```python
from build123d import *

# Parameters (mm, degrees)
SKETCH1_W           = 101.4
SKETCH1_H           = 92.5
SKETCH1_R           = 1.5
SKETCH1_R_2         = 2
BOSS_EXTRUDE1_DEPTH = 10


with BuildPart() as part:
    # Sketch1 → Boss-Extrude1 (new body)
    with BuildSketch(Plane(origin=(0, 0, 0), x_dir=(1, 0, 0), z_dir=(0, 1, 0))):
        Rectangle(SKETCH1_W, SKETCH1_H)
        with Locations((-40, 42.75)):
            Circle(SKETCH1_R, mode=Mode.SUBTRACT)
        with Locations((-20, 42.75)):
            Circle(SKETCH1_R, mode=Mode.SUBTRACT)
        with Locations((-20, 17.75)):
            Circle(SKETCH1_R, mode=Mode.SUBTRACT)
        with Locations((-40, 17.75)):
            Circle(SKETCH1_R, mode=Mode.SUBTRACT)
        with Locations((-40, -42.75)):
            Circle(SKETCH1_R, mode=Mode.SUBTRACT)
        with Locations((-20, -42.75)):
            Circle(SKETCH1_R, mode=Mode.SUBTRACT)
        with Locations((-20, -17.75)):
            Circle(SKETCH1_R, mode=Mode.SUBTRACT)
        with Locations((-40, -17.75)):
            Circle(SKETCH1_R, mode=Mode.SUBTRACT)
        with Locations((40, -17.75)):
            Circle(SKETCH1_R, mode=Mode.SUBTRACT)
        with Locations((20, -17.75)):
            Circle(SKETCH1_R, mode=Mode.SUBTRACT)
        with Locations((20, -42.75)):
            Circle(SKETCH1_R, mode=Mode.SUBTRACT)
        with Locations((40, -42.75)):
            Circle(SKETCH1_R, mode=Mode.SUBTRACT)
        with Locations((40, 17.75)):
            Circle(SKETCH1_R, mode=Mode.SUBTRACT)
        with Locations((20, 17.75)):
            Circle(SKETCH1_R, mode=Mode.SUBTRACT)
        with Locations((20, 42.75)):
            Circle(SKETCH1_R, mode=Mode.SUBTRACT)
        with Locations((40, 42.75)):
            Circle(SKETCH1_R, mode=Mode.SUBTRACT)
        with Locations((-30, 32.5)):
            Circle(SKETCH1_R_2, mode=Mode.SUBTRACT)
        with Locations((30, 32.5)):
            Circle(SKETCH1_R_2, mode=Mode.SUBTRACT)
        with Locations((30, -32.5)):
            Circle(SKETCH1_R_2, mode=Mode.SUBTRACT)
        with Locations((-30, -32.5)):
            Circle(SKETCH1_R_2, mode=Mode.SUBTRACT)
    extrude(amount=BOSS_EXTRUDE1_DEPTH)


solid = part.part
```
Geometry check sheet. Reference: the model listing, model coordinates, mm. Round coordinates to 2 decimals unless told otherwise and drop trailing zeros. Order: outer loops, then holes, each group sorted by start corner. A loop starts at its lowest first (then second) coordinate and runs counter-clockwise, first axis right, second up. Notation, with made-up numbers: (76.25, 76.5) - (86.25, 76.5) arc R14 ccw to (86.25, 96.5) - close; hole circle Ø8 at (-12.75, 34.5). An arc over 180 degrees is marked (long way). Use a Markdown table: item, result. Add a question column.
1) Section check C-C (y = 8.25). Count the separate pieces of the cut face and the enclosed holes in it, then the cut area to 3 significant figures.
2) Mould release check, pull along X, two halves, no side actions. Record for faces 1 (the cylindrical face through (-41.19, 4.93, 43.66)), 2 (the flat face through (-1, 5, 46.25)), 3 (the flat face through (50.7, 5, 1)), 4 (the cylindrical face through (-41.19, 4.93, -41.84)): released by +X, released by -X, zero draft, split by the parting line, or undercut.
3) Section check A-A (x = -30). Record the cut outline in (y, z).
4) Section check D-D (z = 17.75). Record the cut outline in (x, y).
5) Section check B-B (z = 32.5). Record the cut outline in (x, y).
6) Thickness scan on line 1 along X through (y, z) = (4.5, 32.5); line 2 along X through (y, z) = (4.5, 42.75); line 3 along Z through (x, y) = (-30, 4). Record the ranges inside material, lowest first.
Established:
| question | item | result |
|---|---|---|
| 1 | separate pieces | 1 |
| 1 | enclosed holes | 20 |
| 1 | area | 9,220 mm2 |
| 2 | face 1 | undercut |
| 2 | face 2 | zero draft |
| 2 | face 3 | released by +X |
| 2 | face 4 | undercut |
| 3 | outline | (0, -46.25) - (10, -46.25) - (10, -34.5) - (0, -34.5) - close; (0, -30.5) - (10, -30.5) - (10, 30.5) - (0, 30.5) - close; (0, 34.5) - (10, 34.5) - (10, 46.25) - (0, 46.25) - close |
| 4 | outline | (-50.7, 0) - (-41.5, 0) - (-41.5, 10) - (-50.7, 10) - close; (-38.5, 0) - (-21.5, 0) - (-21.5, 10) - (-38.5, 10) - close; (-18.5, 0) - (18.5, 0) - (18.5, 10) - (-18.5, 10) - close; (21.5, 0) - (38.5, 0) - (38.5, 10) - (21.5, 10) - close; (41.5, 0) - (50.7, 0) - (50.7, 10) - (41.5, 10) - close |
| 5 | outline | (-50.7, 0) - (-32, 0) - (-32, 10) - (-50.7, 10) - close; (-28, 0) - (28, 0) - (28, 10) - (-28, 10) - close; (32, 0) - (50.7, 0) - (50.7, 10) - (32, 10) - close |
| 6 | line 1 | -50.7 to -32, -28 to 28, 32 to 50.7 |
| 6 | line 2 | -50.7 to -41.5, -38.5 to -21.5, -18.5 to 18.5, 21.5 to 38.5, 41.5 to 50.7 |
| 6 | line 3 | -46.25 to -34.5, -30.5 to 30.5, 34.5 to 46.25 |
